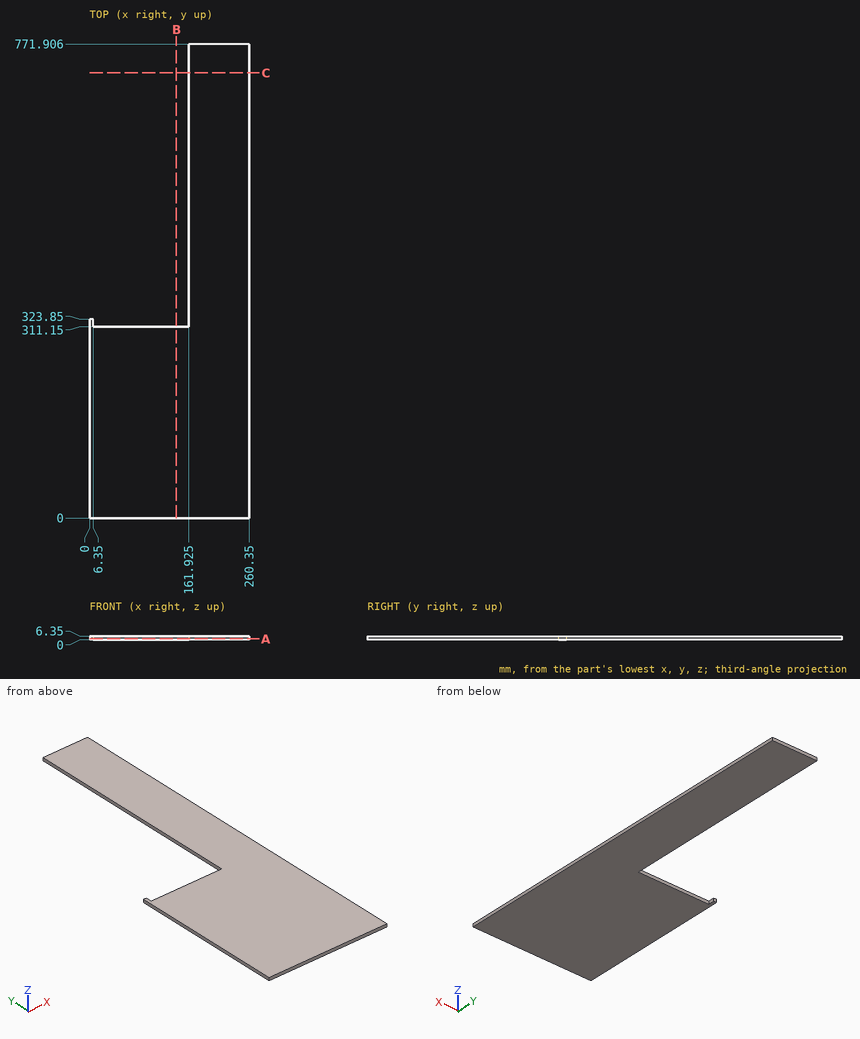
Verification items for this drawing (mm, ordinates from the low corner). Give positions to 0.01 mm unless a question says otherwise; leave off trailing zeros. Write each loop counter-clockwise with the first axis right and the second up, starting at its lowest first coordinate (ties: lowest second). Pieces come first, ordered by that corner, then holes. Notation, with made-up numbers: (17.5, 44.5) -> (71.5, 44.5) arc R9 cw to (71.5, 60.5) -> close; hole circle Ø11 at (70.5, 20.5). An arc over 180 degrees is marked (long way). Use one line per item in the form item = value.
Item 1: Depth check by flat-ended pin: pin 1 Ø3 at (x, z) = (3.5, 3) entering from +Y; pin 2 Ø3 at (y, z) = (407, 1) entering from -X (3 decimals). Enter the tip coordinate at first touch or a pass-through.
Results list:
pin_1 = 323.85
pin_2 = 161.925
Item 2: Sectioned sample at C-C on y = 725. Enter the section's corners in (x, z) (3 decimals), plus the area to 3 significant figures.
Results list:
outline = (161.925, 0) -> (260.35, 0) -> (260.35, 6.35) -> (161.925, 6.35) -> close
area = 625 mm2
Item 3: Sectioned sample at B-B on x = 141.5. Enter the section's corners in (y, z).
Results list:
outline = (0, 0) -> (311.15, 0) -> (311.15, 6.35) -> (0, 6.35) -> close
Item 4: Scan lines: line 1 (X direction, y = 482.5, z = 5.25) (3 decimals); line 2 (Y direction, x = 128.5, z = 1.25). Record each from-to range of solid material in increasing order.
Results list:
line_1 = 161.925 to 260.35
line_2 = 0 to 311.15
Item 5: Sectioned sample at A-A on z = 2. Enter the section's corners in (x, y) (3 decimals), plus the area to 3 significant figures.
Results list:
outline = (0, 0) -> (260.35, 0) -> (260.35, 771.906) -> (161.925, 771.906) -> (161.925, 311.15) -> (6.35, 311.15) -> (6.35, 323.85) -> (0, 323.85) -> close
area = 126,000 mm2
